from build123d import *

# Parameters (mm, degrees)
BOX030_W                             = 48
BOX030_H                             = 60
BOX030_DEPTH                         = 10
BOX028_W                             = 2.6
BOX028_H                             = 10.6
BOX028_DEPTH                         = 15
BOX027_W                             = 2.6
BOX027_H                             = 10.6
BOX027_DEPTH                         = 15
EXTRUDE076_DEPTH                     = 34.5
EXTRUDE076_ONTO_SKETCH082_ROLL_ANGLE = 90
EXTRUDE075_DEPTH                     = 34.5
EXTRUDE075_ONTO_SKETCH081_ROLL_ANGLE = 90
EXTRUDE077_DEPTH                     = 10.5
EXTRUDE077_ONTO_SKETCH083_ROLL_ANGLE = 90
EXTRUDE080_DEPTH                     = 100
EXTRUDE079_DEPTH                     = 2
EXTRUDE079_ONTO_SKETCH085_ROLL_ANGLE = 90
BOX029_W                             = 80
BOX029_H                             = 28
BOX029_DEPTH                         = 30
EXTRUDE078_DEPTH                     = 35.5
EXTRUDE078_ONTO_SKETCH084_ROLL_ANGLE = 90
BOX032_W                             = 48
BOX032_H                             = 60
BOX032_DEPTH                         = 35
BOX031_W                             = 48
BOX031_H                             = 60
BOX031_DEPTH                         = 35
BOX033_W                             = 48
BOX033_H                             = 60
BOX033_DEPTH                         = 35
EXTRUDE081_DEPTH                     = 2
EXTRUDE081_ONTO_SKETCH087_ROLL_ANGLE = 90


with BuildPart() as cube:
    # Box030 → Box030 (new body)
    with BuildSketch(Plane(origin=(11, 60.5, -2.6), x_dir=(1, 0, 0), z_dir=(0, 0, 1))):
        with Locations((24, 30)):
            Rectangle(BOX030_W, BOX030_H)
    extrude(amount=BOX030_DEPTH)


with BuildPart() as control_cutout_rec003:
    # Box028 → Box028 (new body)
    with BuildSketch(Plane(origin=(57, 93, 9), x_dir=(1, 0, 0), z_dir=(0, 0, 1))):
        with Locations((1.3, 5.3)):
            Rectangle(BOX028_W, BOX028_H)
    extrude(amount=BOX028_DEPTH)


with BuildPart() as button_cutouts_rec001:
    # Box027 → Box027 (new body)
    with BuildSketch(Plane(origin=(8.3, 93, 9), x_dir=(1, 0, 0), z_dir=(0, 0, 1))):
        with Locations((1.3, 5.3)):
            Rectangle(BOX027_W, BOX027_H)
    extrude(amount=BOX027_DEPTH)

    # Fusion041: union control_cutout_rec003
    add(control_cutout_rec003.part)


with BuildPart() as obj1:
    # Sketch082 as drawn → Extrude076 (new)
    with BuildSketch(Plane.XY):
        Polygon((14, 17), (-5.5, 17), (-5.5, 25.6), (73.5, 25.6), (73.5, 17), (54, 17), (49, 6.7), (49, 6.6), (19, 6.6), (19, 6.7), align=None)
    extrude(amount=-EXTRUDE076_DEPTH)


with BuildPart() as obj1_1:
    # Extrude076 onto Sketch082 roll: moved
    add(obj1.part.rotate(Axis((0, 0, 0), (1, 0, 0)), EXTRUDE076_ONTO_SKETCH082_ROLL_ANGLE))


with BuildPart() as obj1_2:
    # Extrude076 onto Sketch082 placement: moved
    add(obj1_1.part.moved(Location((0, 86, 0))))


with BuildPart() as screen_frame002:
    # Sketch081 as drawn → Extrude075 (new)
    with BuildSketch(Plane.XY):
        with BuildLine():
            Line((-2.5, 14.2), (-2.5, 10.6))
            Line((-2.5, 10.6), (1.6, 10.6))
            Line((1.6, 10.6), (1.6, 11.6))
            Line((1.6, 11.6), (13.6, 11.6))
            Line((13.6, 11.6), (17.6, 7))
            Line((17.6, 7), (50.4, 7))
            Line((50.4, 7), (54.4, 11.1))
            Line((54.4, 11.1), (66.4, 11.1))
            Line((66.4, 11.1), (66.4, 10.6))
            Line((66.4, 10.6), (70.5, 10.6))
            Line((70.5, 10.6), (70.5, 14.2))
            ThreePointArc((70.5, 14.2), (67.863961, 20.563961), (61.5, 23.2))
            Line((6.5, 23.2), (61.5, 23.2))
            ThreePointArc((6.5, 23.2), (0.136039, 20.563961), (-2.5, 14.2))
        make_face()
    extrude(amount=-EXTRUDE075_DEPTH)


with BuildPart() as screen_frame002_1:
    # Extrude075 onto Sketch081 roll: moved
    add(screen_frame002.part.rotate(Axis((0, 0, 0), (1, 0, 0)), EXTRUDE075_ONTO_SKETCH081_ROLL_ANGLE))


with BuildPart() as screen_frame002_2:
    # Extrude075 onto Sketch081 placement: moved
    add(screen_frame002_1.part.moved(Location((0, 86, 0))))

    # Cut031: cut obj1
    add(obj1_2.part, mode=Mode.SUBTRACT)


with BuildPart() as cut032:
    # Sketch083 as drawn → Extrude077 (new)
    with BuildSketch(Plane.XY):
        Polygon((13.6, 12.2), (17.6, 7.2), (50.4, 7.2), (54.4, 12.2), align=None)
    extrude(amount=-EXTRUDE077_DEPTH)


with BuildPart() as cut032_1:
    # Extrude077 onto Sketch083 roll: moved
    add(cut032.part.rotate(Axis((0, 0, 0), (1, 0, 0)), EXTRUDE077_ONTO_SKETCH083_ROLL_ANGLE))


with BuildPart() as cut032_2:
    # Extrude077 onto Sketch083 placement: moved
    add(cut032_1.part.moved(Location((0, 110, 0))))

    # Fusion042: union screen_frame002
    add(screen_frame002_2.part)

    # Cut032: cut button_cutouts_rec001
    add(button_cutouts_rec001.part, mode=Mode.SUBTRACT)


with BuildPart() as round_cut002:
    # Sketch086 → Extrude080 (new body)
    with BuildSketch(Plane.YZ.offset(-14)):
        with BuildLine():
            Line((100, 23.2), (100, 26.2))
            Line((100, 26.2), (138, 26.2))
            Line((138, 26.2), (138, -11.8))
            Line((138, -11.8), (135, -11.8))
            Line((135, -11.8), (135, -1.8))
            ThreePointArc((135, -1.8), (127.67767, 15.87767), (110, 23.2))
            Line((100, 23.2), (110, 23.2))
        make_face()
    extrude(amount=EXTRUDE080_DEPTH)


with BuildPart() as extrude079:
    # Sketch085 as drawn → Extrude079 (new)
    with BuildSketch(Plane.XY):
        with BuildLine():
            Line((-2.5, 14.2), (-2.5, -4.1))
            ThreePointArc((-2.5, -4.1), (0.136039, -10.463961), (6.5, -13.1))
            Line((6.5, -13.1), (61.5, -13.1))
            ThreePointArc((61.5, -13.1), (67.863961, -10.463961), (70.5, -4.1))
            Line((70.5, -4.1), (70.5, 14.2))
            ThreePointArc((70.5, 14.2), (67.863961, 20.563961), (61.5, 23.2))
            Line((6.5, 23.2), (61.5, 23.2))
            ThreePointArc((6.5, 23.2), (0.136039, 20.563961), (-2.5, 14.2))
        make_face()
    extrude(amount=-EXTRUDE079_DEPTH)


with BuildPart() as extrude079_1:
    # Extrude079 onto Sketch085 roll: moved
    add(extrude079.part.rotate(Axis((0, 0, 0), (1, 0, 0)), EXTRUDE079_ONTO_SKETCH085_ROLL_ANGLE))


with BuildPart() as extrude079_2:
    # Extrude079 onto Sketch085 placement: moved
    add(extrude079_1.part.moved(Location((0, 120, 0))))


with BuildPart() as extrude079_3:
    # Extrude079 placement: moved
    add(extrude079_2.part.moved(Location((0, 0.5, 0))))


with BuildPart() as cube008:
    # Box029 → Box029 (new body)
    with BuildSketch(Plane(origin=(-5, 82, 10.6), x_dir=(1, 0, 0), z_dir=(0, 0, 1))):
        with Locations((40, 14)):
            Rectangle(BOX029_W, BOX029_H)
    extrude(amount=BOX029_DEPTH)


with BuildPart() as shell_upper004:
    # Sketch084 as drawn → Extrude078 (new)
    with BuildSketch(Plane.XY):
        with BuildLine():
            Line((-2.5, 14.2), (-2.5, -4.1))
            ThreePointArc((-2.5, -4.1), (0.136039, -10.463961), (6.5, -13.1))
            Line((6.5, -13.1), (61.5, -13.1))
            ThreePointArc((61.5, -13.1), (67.863961, -10.463961), (70.5, -4.1))
            Line((70.5, -4.1), (70.5, 14.2))
            ThreePointArc((70.5, 14.2), (67.863961, 20.563961), (61.5, 23.2))
            Line((6.5, 23.2), (61.5, 23.2))
            ThreePointArc((6.5, 23.2), (0.136039, 20.563961), (-2.5, 14.2))
        make_face()
        with BuildLine():
            Line((1.6, 1.2), (-1, 1.2))
            Line((-1, 1.2), (-1, -0.1))
            Line((-1, -0.1), (1.6, -0.1))
            Line((1.6, -0.1), (1.6, -6.1))
            ThreePointArc((1.6, -6.1), (3.064466, -9.635534), (6.6, -11.1))
            Line((6.6, -11.1), (61.4, -11.1))
            ThreePointArc((61.4, -11.1), (64.935534, -9.635534), (66.4, -6.1))
            Line((66.4, -0.1), (66.4, -6.1))
            Line((69, -0.1), (66.4, -0.1))
            Line((69, 1.2), (69, -0.1))
            Line((66.4, 1.2), (69, 1.2))
            Line((66.4, 5.4), (66.4, 1.2))
            Line((64.4, 5.4), (66.4, 5.4))
            Line((64.4, 7.4), (64.4, 5.4))
            Line((66.4, 7.4), (64.4, 7.4))
            Line((66.4, 10.6), (66.4, 7.4))
            Line((66.4, 10.6), (66.4, 10.8))
            Line((66.4, 10.8), (64.5, 10.8))
            Line((64.5, 10.8), (3.5, 10.8))
            Line((1.6, 10.8), (3.5, 10.8))
            Line((1.6, 10.6), (1.6, 10.8))
            Line((1.6, 10.6), (1.6, 7.4))
            Line((1.6, 7.4), (3.5, 7.4))
            Line((3.5, 7.4), (1.6, 1.2))
        make_face(mode=Mode.SUBTRACT)
    extrude(amount=EXTRUDE078_DEPTH)


with BuildPart() as shell_upper004_1:
    # Extrude078 onto Sketch084 roll: moved
    add(shell_upper004.part.rotate(Axis((0, 0, 0), (1, 0, 0)), EXTRUDE078_ONTO_SKETCH084_ROLL_ANGLE))


with BuildPart() as shell_upper004_2:
    # Extrude078 onto Sketch084 placement: moved
    add(shell_upper004_1.part.moved(Location((0, 120, 0))))


with BuildPart() as shell_upper004_3:
    # Extrude078 placement: moved
    add(shell_upper004_2.part.moved(Location((0, 1.5, 0))))

    # Cut033: cut Cube008
    add(cube008.part, mode=Mode.SUBTRACT)

    # Fusion043: union Extrude079
    add(extrude079_3.part)

    # Cut034: cut round_cut002
    add(round_cut002.part, mode=Mode.SUBTRACT)

    # Fusion044: union Cut032
    add(cut032_2.part)


with BuildPart() as cube010:
    # Box032 → Box032 (new body)
    with BuildSketch(Plane(origin=(54, 60.5, -20.6), x_dir=(1, 0, 0), z_dir=(0, 0, 1))):
        with Locations((24, 30)):
            Rectangle(BOX032_W, BOX032_H)
    extrude(amount=BOX032_DEPTH)


with BuildPart() as cube009:
    # Box031 → Box031 (new body)
    with BuildSketch(Plane(origin=(-33, 60.5, -21.6), x_dir=(1, 0, 0), z_dir=(0, 0, 1))):
        with Locations((24, 30)):
            Rectangle(BOX031_W, BOX031_H)
    extrude(amount=BOX031_DEPTH)


with BuildPart() as fusion045:
    # Box033 → Box033 (new body)
    with BuildSketch(Plane(origin=(11, 60.5, -32.6), x_dir=(1, 0, 0), z_dir=(0, 0, 1))):
        with Locations((24, 30)):
            Rectangle(BOX033_W, BOX033_H)
    extrude(amount=BOX033_DEPTH)

    # Fusion045: union Cube010, Cube009
    add(cube010.part)
    add(cube009.part)


with BuildPart() as shell_upper_tuned:
    # Sketch087 as drawn → Extrude081 (new)
    with BuildSketch(Plane.XY):
        with BuildLine():
            Line((-2.5, 14.2), (-2.5, -4.099997))
            ThreePointArc((-2.5, -4.099997), (0.136039, -10.463958), (6.5, -13.099997))
            Line((6.5, -13.099997), (61.498163, -13.099997))
            ThreePointArc((61.498163, -13.099997), (67.863423, -10.46342), (70.5, -4.09816))
            Line((70.5, -4.09816), (70.5, 14.2))
            ThreePointArc((70.5, 14.2), (67.863961, 20.563961), (61.5, 23.2))
            Line((6.5, 23.2), (61.5, 23.2))
            ThreePointArc((6.5, 23.2), (0.136039, 20.563961), (-2.5, 14.2))
        make_face()
        with BuildLine():
            Line((1.6, 1.200003), (-1, 1.200003))
            Line((-1, 1.200003), (-1, -0.099997))
            Line((-1, -0.099997), (1.6, -0.099997))
            Line((1.6, -0.099997), (1.6, -6.099997))
            ThreePointArc((1.6, -6.099997), (3.064466, -9.635531), (6.6, -11.099997))
            Line((6.6, -11.099997), (61.399986, -11.099997))
            ThreePointArc((61.399986, -11.099997), (64.936819, -9.634993), (66.401823, -6.09816))
            Line((66.401823, -0.09816), (66.401823, -6.09816))
            Line((69, -0.09816), (66.401823, -0.09816))
            Line((69, 1.20184), (69, -0.09816))
            Line((66.401823, 1.20184), (69, 1.20184))
            Line((66.401823, 5.40184), (66.401823, 1.20184))
            Line((64.3846, 5.40184), (66.401823, 5.40184))
            Line((64.3846, 10.90184), (64.3846, 5.40184))
            Line((54.2, 10.90184), (64.3846, 10.90184))
            Line((50.4, 7), (54.2, 10.90184))
            Line((17.6, 7), (50.4, 7))
            Line((14.2, 10.97071), (17.6, 7))
            Line((3.5, 10.97071), (14.2, 10.97071))
            Line((3.5, 7.47071), (3.5, 10.97071))
            Line((3.5, 7.47071), (1.6, 1.200003))
        make_face(mode=Mode.SUBTRACT)
    extrude(amount=-EXTRUDE081_DEPTH)


with BuildPart() as shell_upper_tuned_1:
    # Extrude081 onto Sketch087 roll: moved
    add(shell_upper_tuned.part.rotate(Axis((0, 0, 0), (1, 0, 0)), EXTRUDE081_ONTO_SKETCH087_ROLL_ANGLE))


with BuildPart() as shell_upper_tuned_2:
    # Extrude081 onto Sketch087 placement: moved
    add(shell_upper_tuned_1.part.moved(Location((0, 84, 0))))


with BuildPart() as shell_upper_tuned_3:
    # Extrude081 placement: moved
    add(shell_upper_tuned_2.part.moved(Location((0, 24, 0))))

    # Cut035: cut Fusion045
    add(fusion045.part, mode=Mode.SUBTRACT)

    # Fusion046: union shell_upper004
    add(shell_upper004_3.part)

    # Cut036: cut Cube
    add(cube.part, mode=Mode.SUBTRACT)


solid = shell_upper_tuned_3.part
Here's how the part is built. I have some questions about the finished solid (model axes, mm). A direction names the side the tool comes from. Round coordinates to 2 decimals unless told otherwise and drop trailing zeros. Order: outer loops, then holes, each group sorted by start corner. A loop starts at its lowest first (then second) coordinate and runs counter-clockwise, first axis right, second up. Notation, with made-up numbers: (71.25, 86.25) -> (100.25, 86.25) arc R30 ccw to (100.25, 116.25) -> close; hole circle Ø3 at (-9, 67.5). An arc over 180 degrees is marked (long way). Return JSON: item names as keys, results as strings.
Q1. For pin 1 Ø2 at (x, y) = (0, 97.5) entering from -Z; pin 2 Ø6.5 at (x, z) = (31.5, 4) entering from -Y; pin 3 Ø12.5 at (x, z) = (25.5, 16) entering from -Y, each with a flat end and sliding along its axis, tell me the tip position at first contact or that it passes through.
Filled sheet:
{"pin 1": "stops at z = -11.22", "pin 2": "stops at y = 120.5", "pin 3": "stops at y = 108"}
Q2. I need wall thicknesses on line 1 along Z through (x, y) = (55, 98.5); line 2 along X through (y, z) = (115.5, 10); line 3 along Z through (x, y) = (65, 107). Which ranges of each line are inside material? Lowest first, please. Write a range as from..to.
Filled sheet:
{"line 1": "z = -13.1..-11.1, 11.1..17", "line 2": "x = -2.5..1.6, 14.99..53.33, 66.4..70.5", "line 3": "z = -12.39..-9.57, 5.4..7.4, 11.1..17"}
Q3. If we section it at A-A on x = 28.5: List the corners of the cut face in (y, z) for me.
Filled sheet:
{"outline": "(86, -13.1) -> (122.5, -13.1) -> (122.5, 19.85) arc R25 ccw to (110, 23.2) -> (108, 23.2) -> (108, 7.4) -> (120.5, 7.4) -> (120.5, -11.1) -> (86, -11.1) -> close"}
Q4. If we section it at C-C on z = 2.5: List the corners of the cut face in (x, y) for me.
Filled sheet:
{"outline": "(-2.5, 86) -> (2, 86) -> (2, 120.5) -> (66.4, 120.5) -> (66.4, 86) -> (70.5, 86) -> (70.5, 122.5) -> (-2.5, 122.5) -> close"}
Q5. If we section it at D-D on y = 100: Give the number of separate pieces and of enclosed holes in the cut face, plus the area to 3 significant figures.
Filled sheet:
{"separate pieces": "3", "enclosed holes": "0", "area": "499 mm^2"}
Q6. Which directions (+Z, -Z, +X, -X, +Y, -Y) give clear straight access to the entire face, cutting with the end or side of a thin tool? Please do faces 1 (the flat face through (66.4, 103, 9)), 2 (the flat face through (51.703, 96.846, 12.267)), 3 (the flat face through (62, 97, 17)), 4 (the flat face through (58, 93, 14)).
Filled sheet:
{"face 1": "-Y", "face 2": "+Z, -Y", "face 3": "+Z, +X, -X, -Y", "face 4": "+Z"}
Q7. If we mould it in two halves opening along Z, with no side actions, what happens to faces 5 (the flat face through (34, 104, -13.1)), 6 (the flat face through (70.5, 104, 5)), 7 (the flat face through (66.4, 103, 3))? For each: released by +Z, released by -Z, zero draft, split by the parting line, or undercut.
Filled sheet:
{"face 5": "released by -Z", "face 6": "zero draft", "face 7": "undercut"}
